Can you work these out from the model? Positions are in its coordinate system, mm. Face numbers are marked on the shaded views. A direction names the side the tool comes from. Round coordinates to 2 decimals unless told otherwise and drop trailing zeros. Use a Markdown table: item, result. Add a question column.
Q1. I need wall thicknesses on line 1 along Z through (x, y) = (-1.75, 141); line 2 along Y through (x, z) = (-1.75, -528); line 3 along Z through (x, y) = (7, 165). Which ranges of each line are inside material? Lowest first, please. Write a range as [from, to].
Q2. For the marked faces 1 and 2, which set-ups out of +Z, -Z, +X, -X, +Y, -Y let a thin tool reach every point of the face, with its end or its side?
Q3. I'm going to push flat-ended pins straight in: pin 1 Ø6 at (x, y) = (3, 251) entering from +Z; pin 2 Ø1.2 at (x, z) = (3, -474.5) entering from -Y; pin 3 Ø4 at (x, z) = (5, -510) entering from -Y. Where does each tip first touch, or does it pass through?
Q4. We'd pull the mould along Y, two halves only. Please class the marked faces 3, 4 and 5: +Y half, -Y half, draft (parallel to the pull), parting line (faces both ways), or undercut.
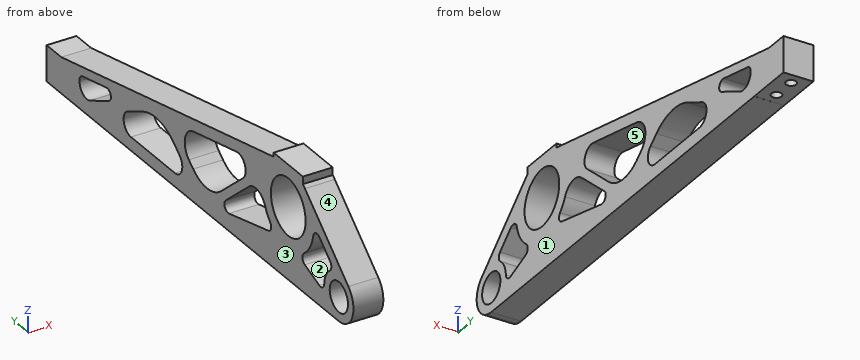
```python
from build123d import *

# Parameters (mm, degrees)
SKETCH1_R                       = 15.08125
SKETCH1_R_2                     = 7.9375
BOSS_EXTRUDE1_DEPTH             = 7.9375
TAP_DRILL_FOR_1_4_28_TAP1_D     = 5.4102
TAP_DRILL_FOR_1_4_28_TAP1_DEPTH = 14.249611939
TAP_DRILL_FOR_1_4_28_TAP1_TIP   = 1.625388061


with BuildPart() as part:
    # Sketch1 → Boss-Extrude1 (new body, symmetric)
    with BuildSketch(Plane(origin=(0, 0, 0), x_dir=(0, 0, -1), z_dir=(1, 0, 0))):
        with BuildLine():
            ThreePointArc((477.273006468, 55.573710947), (477.957555138, 54.643144528), (478.689532564, 53.74940531))
            Line((478.689532564, 53.74940531), (511.29915841, 15.980017214))
            ThreePointArc((511.29915841, 15.980017214), (525.339576994, 12.376406632), (533.611992871, 24.279620434))
            Line((533.611992871, 24.279620434), (533.611992871, 252.869620434))
            ThreePointArc((533.611992871, 252.869620434), (533.621992871, 252.879620434), (533.611992871, 252.889620434))
            Line((533.611992871, 252.889620434), (533.611992871, 278.279620434))
            Line((533.611992871, 278.279620434), (514.561992871, 278.279620434))
            Line((514.561992871, 278.279620434), (514.561992871, 265.579620434))
            Line((514.561992871, 265.579620434), (475.482925659, 80.973710947))
            Line((475.482925659, 80.973710947), (473.286992871, 80.973710947))
            Line((473.286992871, 80.973710947), (473.286992871, 55.573710947))
            Line((473.286992871, 55.573710947), (477.273006468, 55.573710947))
        make_face()
        with Locations((495.511992871, 68.273710947)):
            Circle(SKETCH1_R, mode=Mode.SUBTRACT)
        with BuildLine():
            Line((513.492352541, 154.682917565), (516.491551882, 150.932886553))
            ThreePointArc((516.491551882, 150.932886553), (520.662032348, 138.733869971), (516.108721588, 126.672515404))
            Line((516.108721588, 126.672515404), (499.792202262, 107.541452006))
            ThreePointArc((499.792202262, 107.541452006), (492.156570852, 105.964813857), (488.748431965, 112.977177526))
            Line((488.748431965, 112.977177526), (496.735281949, 150.706320271))
            ThreePointArc((496.735281949, 150.706320271), (503.854492534, 158.001314948), (513.492352541, 154.682917565))
        make_face(mode=Mode.SUBTRACT)
        with BuildLine():
            Line((505.940679161, 31.90308853), (497.871284255, 41.249289229))
            ThreePointArc((497.871284255, 41.249289229), (497.275971755, 44.367979343), (499.679180371, 46.442880148))
            ThreePointArc((499.679180371, 46.442880148), (507.170500261, 49.352034741), (513.137493678, 54.73516057))
            ThreePointArc((513.137493678, 54.73516057), (516.142098705, 55.938560413), (518.64094789, 53.8814811))
            Line((518.64094789, 53.8814811), (523.222631148, 41.220667502))
            ThreePointArc((523.222631148, 41.220667502), (522.874411989, 38.372433477), (520.372083072, 36.968138764))
            ThreePointArc((520.372083072, 36.968138764), (515.06938347, 35.555874927), (510.857508795, 32.038315555))
            ThreePointArc((510.857508795, 32.038315555), (508.431176446, 30.804189453), (505.940679161, 31.90308853))
        make_face(mode=Mode.SUBTRACT)
        with Locations((520.911992871, 24.279620434)):
            Circle(SKETCH1_R_2, mode=Mode.SUBTRACT)
        with BuildLine():
            ThreePointArc((518.944357913, 122.658172896), (522.790818804, 123.432213046), (524.452355406, 119.877822007))
            Line((524.452355406, 119.877822007), (516.472291206, 85.606211423))
            ThreePointArc((516.472291206, 85.606211423), (514.260132633, 83.275664888), (511.146510795, 84.069674807))
            ThreePointArc((511.146510795, 84.069674807), (508.195718311, 86.524018724), (504.866661886, 88.434087744))
            ThreePointArc((504.866661886, 88.434087744), (499.826228678, 94.721972649), (501.785115668, 102.539019742))
            Line((501.785115668, 102.539019742), (518.944357913, 122.658172896))
        make_face(mode=Mode.SUBTRACT)
        with BuildLine():
            ThreePointArc((526.468242871, 166.731606566), (522.219734771, 160.739425678), (515.159193487, 162.76545866))
            Line((515.159193487, 162.76545866), (511.105468766, 167.834009193))
            ThreePointArc((511.105468766, 167.834009193), (505.69956043, 180.870864765), (508.086772693, 194.780741319))
            Line((508.086772693, 194.780741319), (514.404519469, 207.809941801))
            ThreePointArc((514.404519469, 207.809941801), (521.5395726, 211.228293635), (526.468242871, 205.039406675))
            Line((526.468242871, 205.039406675), (526.468242871, 166.731606566))
        make_face(mode=Mode.SUBTRACT)
        with BuildLine():
            ThreePointArc((515.536548916, 247.187161956), (516.643598283, 248.996229375), (518.642714422, 249.704620434))
            Line((518.642714422, 249.704620434), (519.289846204, 249.704620434))
            ThreePointArc((519.289846204, 249.704620434), (524.671082031, 246.725792482), (525.003569607, 240.584085308))
            Line((525.003569607, 240.584085308), (517.071165151, 224.224947846))
            ThreePointArc((517.071165151, 224.224947846), (513.18532078, 222.606581), (511.108137945, 226.26775693))
            Line((511.108137945, 226.26775693), (515.536548916, 247.187161956))
        make_face(mode=Mode.SUBTRACT)
    extrude(amount=BOSS_EXTRUDE1_DEPTH, both=True)

    # Tap Drill for 1/4-28 Tap1
    with Locations(Plane(origin=(0, 271.929620434, -533.611992871), x_dir=(-1, 0, 0), z_dir=(0, 0, -1))):
        with Locations((0, 0), (0, -12.7)):
            Hole(TAP_DRILL_FOR_1_4_28_TAP1_D / 2, depth=TAP_DRILL_FOR_1_4_28_TAP1_DEPTH)
            with Locations((0, 0, -(TAP_DRILL_FOR_1_4_28_TAP1_DEPTH + TAP_DRILL_FOR_1_4_28_TAP1_TIP / 2))):  # 118° drill point
                Cone(0, TAP_DRILL_FOR_1_4_28_TAP1_D / 2, TAP_DRILL_FOR_1_4_28_TAP1_TIP, mode=Mode.SUBTRACT)


solid = part.part
```
Answer below:
| question | item | result |
|---|---|---|
| 1 | line 1 | [-533.61, -520.56], [-494.68, -488.19] |
| 1 | line 2 | [13.74, 20.71], [27.85, 257.17], [261.29, 269.87], [273.99, 278.28] |
| 1 | line 3 | [-533.61, -526.23], [-513.37, -493.27] |
| 2 | face 1 | +Z, -Z, +X, +Y, -Y |
| 2 | face 2 | +X, -X |
| 3 | pin 1 | z = -510.84 |
| 3 | pin 2 | y = 55.57 |
| 3 | pin 3 | y = 15.23 |
| 4 | face 3 | draft |
| 4 | face 4 | -Y half |
| 4 | face 5 | undercut |
